Read the model definition and answer for the solid it produces. Units are mm, in the model's axes. A direction names the side the tool comes from. Coordinates: 2 decimals unless noted, no trailing zeros. Loops run counter-clockwise (first coordinate to the right, second up) from the corner with the lowest first, then second, coordinate; pieces in that order, holes last.
from build123d import *

# Parameters (mm, degrees)
SKETCH1_W           = 90
SKETCH1_H           = 90
BOSS_EXTRUDE1_DEPTH = 70
SHELL2_T            = -5
CUT_EXTRUDE1_REACH  = 96.604
SKETCH2_W           = 70
SKETCH2_H           = 24
BOSS_EXTRUDE2_DEPTH = 7
SKETCH5_W           = 40
SKETCH5_H           = 40
CUT_EXTRUDE2_DEPTH  = 2
CUT_EXTRUDE3_REACH  = 95.134
SKETCH6_W           = 2
SKETCH6_H           = 40


with BuildPart() as part:
    # Sketch1 → Boss-Extrude1 (new body)
    with BuildSketch(Plane.XY):
        Rectangle(SKETCH1_W, SKETCH1_H)
    extrude(amount=BOSS_EXTRUDE1_DEPTH)

    # Shell2
    shell2_openings = [part.faces().sort_by_distance(p)[0] for p in [
        (0, 0, 0),
    ]]
    offset(amount=SHELL2_T, openings=shell2_openings, kind=Kind.INTERSECTION)

    # Sketch2 → Cut-Extrude1 (cut, up to next)
    with BuildSketch(Plane.XY.offset(70), mode=Mode.PRIVATE) as cut_extrude1_sk1:
        with Locations((0, 20)):
            Rectangle(SKETCH2_W, SKETCH2_H)
    cut_extrude1_tool1 = extrude(cut_extrude1_sk1.sketch, amount=-CUT_EXTRUDE1_REACH, mode=Mode.PRIVATE) & part.part
    add(cut_extrude1_tool1.solids().sort_by_distance((0, 20, 70))[0], mode=Mode.SUBTRACT)

    # Sketch4 → Boss-Extrude2 (add)
    with BuildSketch(Plane(origin=(0, 0, 65), x_dir=(-1, 0, 0), z_dir=(0, 0, -1))):
        Polygon((-40, 38), (-40, 32), (-35, 32), (35, 32), (35, 8), (-35, 8), (-40, 8), (-40, 2), (40, 2), (40, 38), align=None)
    extrude(amount=BOSS_EXTRUDE2_DEPTH)

    # Sketch5 → Cut-Extrude2 (cut)
    with BuildSketch(Plane.XY.offset(70)):
        with Locations((0, -18)):
            Rectangle(SKETCH5_W, SKETCH5_H)
    extrude(amount=-CUT_EXTRUDE2_DEPTH, mode=Mode.SUBTRACT)

    # Sketch6 → Cut-Extrude3 (cut, up to next)
    with BuildSketch(Plane.XY.offset(68), mode=Mode.PRIVATE) as cut_extrude3_sk1:
        with Locations((-19, -18)):
            Rectangle(SKETCH6_W, SKETCH6_H)
    cut_extrude3_tool1 = extrude(cut_extrude3_sk1.sketch, amount=-CUT_EXTRUDE3_REACH, mode=Mode.PRIVATE) & part.part
    add(cut_extrude3_tool1.solids().sort_by_distance((-19, -18, 68))[0], mode=Mode.SUBTRACT)


solid = part.part
Item 1: A cutting plane is placed at D-D on z = 12. Determine the outline of the cut face in (x, y), then the cut area to 3 significant figures.
Numbers:
outline: (-45, -45) - (45, -45) - (45, 45) - (-45, 45) - close; hole (-40, -40) - (40, -40) - (40, 40) - (-40, 40) - close
area: 1,700 mm2
Item 2: A cutting plane is placed at A-A on x = -4. Determine the outline of the cut face in (y, z).
Numbers:
outline: (-45, 0) - (-40, 0) - (-40, 65) - (2, 65) - (2, 58) - (8, 58) - (8, 70) - (2, 70) - (2, 68) - (-38, 68) - (-38, 70) - (-45, 70) - close; (32, 58) - (38, 58) - (38, 65) - (40, 65) - (40, 0) - (45, 0) - (45, 70) - (32, 70) - close
Item 3: Find the intervals of material crossed by line 1 along Y through (x, z) = (-14.5, 64); line 2 along Y through (x, z) = (-13, 48.5), in increasing order.
Numbers:
line 1: y = -45 to -40, 2 to 8, 32 to 38, 40 to 45
line 2: y = -45 to -40, 40 to 45
Item 4: A cutting plane is placed at B-B on y = -18. Determine the outline of the cut face in (x, z), then the cut area to 3 significant figures.
Numbers:
outline: (-45, 0) - (-40, 0) - (-40, 65) - (-20, 65) - (-20, 70) - (-45, 70) - close; (-18, 65) - (40, 65) - (40, 0) - (45, 0) - (45, 70) - (20, 70) - (20, 68) - (-18, 68) - close
area: 1,010 mm2
Item 5: A cutting plane is placed at C-C on z = 61.5. Determine the outline of the cut face in (x, y), then the cut area to 3 significant figures.
Numbers:
outline: (-45, -45) - (45, -45) - (45, 45) - (-45, 45) - close; hole (-40, -40) - (40, -40) - (40, 2) - (-40, 2) - close; hole (-40, 38) - (40, 38) - (40, 40) - (-40, 40) - close; hole (-35, 8) - (40, 8) - (40, 32) - (-35, 32) - close
area: 2,780 mm2
Item 6: Given pin 1 (1.5 mm diameter, centred on x = -25.5, y = 10.5, fed in from +Z); pin 2 (5 mm diameter, centred on x = 24.5, y = -29, fed in from -Z); pin 3 (1 mm diameter, centred on x = -2, y = -16, fed in from +Z), each flat-ended and moving along its own axis, determine where each tip first touches the part or whether it passes through.
Numbers:
pin 1: passes through
pin 2: stops at z = 65
pin 3: stops at z = 68
Item 7: Which of the six approach directions +Z, -Z, +X, -X, +Y, -Y give full straight-line access (tool end or side, diameter ignored) to faces 1 (the face through (0, -38, 69)), 2 (the face through (-40.2, 6.9, 0)), 3 (the face through (1, 2, 63)), 4 (the face through (35, 20, 68)), 5 (the face through (40, -1, 32))?
Numbers:
face 1: +Z
face 2: -Z, +X, -X, +Y, -Y
face 3: none
face 4: +Z, -Z
face 5: -Z
